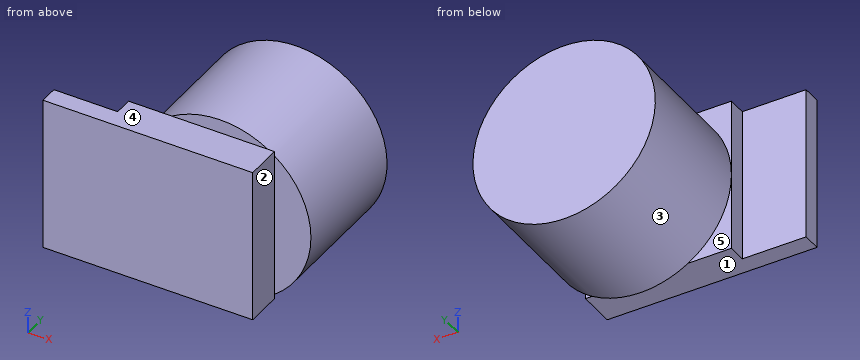
```python
from build123d import *

# Parameters (mm, degrees)
SKETCH1_W           = 11.5
SKETCH1_H           = 8.5
BOSS_EXTRUDE1_DEPTH = 2
SKETCH2_R           = 5
BOSS_EXTRUDE2_DEPTH = 7
SKETCH3_W           = 3.5
SKETCH3_H           = 8.5
CUT_EXTRUDE1_DEPTH  = 1


with BuildPart() as part:
    # Sketch1 → Boss-Extrude1 (new body)
    with BuildSketch(Plane(origin=(0, 0, 0), x_dir=(1, 0, 0), z_dir=(0, 1, 0))):
        Rectangle(SKETCH1_W, SKETCH1_H)
    extrude(amount=BOSS_EXTRUDE1_DEPTH)

    # Sketch2 → Boss-Extrude2 (add)
    with BuildSketch(Plane(origin=(0, 2, 0), x_dir=(1, 0, 0), z_dir=(0, 1, 0))):
        with Locations(Location((2.75, 0, 0), (0, 0, 58.211669383))):
            Circle(SKETCH2_R)
    extrude(amount=BOSS_EXTRUDE2_DEPTH)

    # Sketch3 → Cut-Extrude1 (cut)
    with BuildSketch(Plane(origin=(0, 2, 0), x_dir=(1, 0, 0), z_dir=(0, 1, 0))):
        with Locations((-4, 0)):
            Rectangle(SKETCH3_W, SKETCH3_H)
    extrude(amount=-CUT_EXTRUDE1_DEPTH, mode=Mode.SUBTRACT)


solid = part.part
```
Geometry: final body of the model. Coordinates: model frame, mm. Face numbers are marked on the shaded views. A direction names the side the tool comes from. Round coordinates to 2 decimals unless told otherwise and drop trailing zeros. Order: outer loops, then holes, each group sorted by start corner. A loop starts at its lowest first (then second) coordinate and runs counter-clockwise, first axis right, second up. Notation, with made-up numbers: (59, -29.75) -> (74, -29.75) arc R23 ccw to (74, 4.25) -> close; hole circle Ø5 at (33, 63.25). An arc over 180 degrees is marked (long way). Write each question's results on one line, items separated by ' | '.
Q1. Access query for the marked faces 1, 2, 3, 4 and 5. Directions: +Z, -Z, +X, -X, +Y, -Y. A direction counts if a zero-diameter tool reaches every point of the face in a straight line with its end or side. Return the directions, or none.
Response values:
face 1: -Z, +X, -X, -Y | face 2: +Z, -Z, +X, -Y | face 3: +Y | face 4: +Z, +X, -X, -Y | face 5: -Z, -X, +Y
Q2. Section query D-D (z = -1). Output: boundary loops of the cut face in (x, y).
Response values:
outline: (-5.75, 0) -> (5.75, 0) -> (5.75, 2) -> (7.65, 2) -> (7.65, 9) -> (-2.15, 9) -> (-2.15, 2) -> (-2.25, 2) -> (-2.25, 1) -> (-5.75, 1) -> close
Q3. Section query B-B (z = -3.75). Output: boundary loops of the cut face in (x, y).
Response values:
outline: (-5.75, 0) -> (5.75, 0) -> (5.75, 2) -> (6.06, 2) -> (6.06, 9) -> (-0.56, 9) -> (-0.56, 2) -> (-2.25, 2) -> (-2.25, 1) -> (-5.75, 1) -> close
Q4. Section query A-A (x = 2.75). Output: boundary loops of the cut face in (y, z), and give its area (3 significant figures).
Response values:
outline: (0, -4.25) -> (2, -4.25) -> (2, -5) -> (9, -5) -> (9, 5) -> (2, 5) -> (2, 4.25) -> (0, 4.25) -> close | area: 87.0 mm²
Q5. Ray query, line 1 along Y through (x, z) = (6.5, 1.75); line 2 along Y through (x, z) = (-3.75, 3.75); line 3 along Z through (x, y) = (4.5, 1.75). Return the intervals inside material, ascending.
Response values:
line 1: 2 to 9 | line 2: 0 to 1 | line 3: -4.25 to 4.25
Q6. Pin query (flat end, axial travel): pin 1 Ø0.6 at (x, y) = (1.5, 1) entering from -Z; pin 2 Ø2 at (x, y) = (6.5, 6) entering from -Z; pin 3 Ø1 at (x, y) = (-2.5, 0.5) entering from +Z. Return the tip coordinate at first contact, or that it passes through.
Response values:
pin 1: z = -4.25 | pin 2: z = -4.18 | pin 3: z = 4.25
Q7. Section query C-C (y = 8). Output: boundary loops of the cut face in (x, z), and give its area (3 significant figures).
Response values:
outline: circle Ø10 at (2.75, 0) | area: 78.5 mm²
